For this review, take the finished solid that the model builds, in its own axes (mm). A direction names the side the tool comes from. Coordinates: 2 decimals unless noted, no trailing zeros. Loops run counter-clockwise (first coordinate to the right, second up) from the corner with the lowest first, then second, coordinate; pieces in that order, holes last. Notation, with made-up numbers: (54.5, 72) -> (112.5, 72) arc R16 ccw to (112.5, 100) -> close; hole circle Ø3 at (79.25, 32.5). An arc over 180 degrees is marked (long way). Use a Markdown table: item, result.
from build123d import *

# Parameters (mm, degrees)
F1_DEPTH = 225
F3_D     = 8
F5_D     = 5.9


with BuildPart() as f1:
    # F0 (on Front) → F1 (new body, symmetric)
    with BuildSketch(Plane.XZ):
        Polygon((-22.5, -22.5), (22.5, -22.5), (22.5, -18.5), (-18.5, -18.5), (-18.5, 22.5), (-22.5, 22.5), align=None)
    extrude(amount=F1_DEPTH, both=True)

    # F3 (through all)
    with Locations(Plane(origin=(-22.5, 0, 0), x_dir=(0, -1, 0), z_dir=(-1, 0, 0))):
        with Locations((-75, 12.5), (-85, -7.5), (-65, -7.5)):
            Hole(F3_D / 2)

    # F5 (through all)
    with Locations(Plane.XY.offset(-18.5)):
        with Locations((-13.5, -170), (16.5, -170), (16.5, -215), (-13.5, -215), (-13.5, 215), (16.5, 215), (16.5, 170), (-13.5, 170)):
            Hole(F5_D / 2)


solid = f1.part
(1) Mouldability with a two-part tool opening along Y and no side actions: class faces 1 (the face through (-20.47, 72.05, 15.2)), 2 (the face through (-20, -225, -10)), 3 (the face through (-18.5, -3, 2)) as pulls with the +Y half, pulls with the -Y half, needs draft (parallel to the pull), parting line crosses it, or undercut.
Found:
| item | result |
|---|---|
| face 1 | undercut |
| face 2 | pulls with the -Y half |
| face 3 | needs draft |
(2) Take a section at B-B on z = 12.5. Write out the cut boundary in (x, y).
Found:
| item | result |
|---|---|
| outline | (-22.5, -225) -> (-18.5, -225) -> (-18.5, 71) -> (-22.5, 71) -> close; (-22.5, 79) -> (-18.5, 79) -> (-18.5, 225) -> (-22.5, 225) -> close |
(3) Take a section at A-A on y = 75. Write out the cut boundary in (x, z).
Found:
| item | result |
|---|---|
| outline | (-22.5, -22.5) -> (22.5, -22.5) -> (22.5, -18.5) -> (-18.5, -18.5) -> (-18.5, 8.5) -> (-22.5, 8.5) -> close; (-22.5, 16.5) -> (-18.5, 16.5) -> (-18.5, 22.5) -> (-22.5, 22.5) -> close |
(4) Take a section at D-D on x = 9.5. Write out the cut boundary in (y, z), plus the area to 3 significant figures.
Found:
| item | result |
|---|---|
| outline | (-225, -22.5) -> (225, -22.5) -> (225, -18.5) -> (-225, -18.5) -> close |
| area | 1,800 mm^2 |
(5) For pin 1 Ø13 at (y, z) = (75, 12.5) entering from +X; pin 2 Ø9.5 at (x, y) = (16.5, 170) entering from +Z, all flat-tipped, find the tip position at first contact; note any pin that passes through.
Found:
| item | result |
|---|---|
| pin 1 | stops at x = -18.5 |
| pin 2 | stops at z = -18.5 |
(6) Take a section at C-C on z = -7.5. Write out the cut boundary in (x, y).
Found:
| item | result |
|---|---|
| outline | (-22.5, -225) -> (-18.5, -225) -> (-18.5, 61) -> (-22.5, 61) -> close; (-22.5, 69) -> (-18.5, 69) -> (-18.5, 81) -> (-22.5, 81) -> close; (-22.5, 89) -> (-18.5, 89) -> (-18.5, 225) -> (-22.5, 225) -> close |
(7) For line 1 along Y through (x, z) = (-13.5, -20.25); line 2 along X through (y, z) = (170, -20.55); line 3 along Z through (x, y) = (-20, 65), list the stretches that pass through material, from the lowest coordinate up.
Found:
| item | result |
|---|---|
| line 1 | y = -225 to -217.95, -212.05 to -172.95, -167.05 to 167.05, 172.95 to 212.05, 217.95 to 225 |
| line 2 | x = -22.5 to -16.45, -10.55 to 13.55, 19.45 to 22.5 |
| line 3 | z = -22.5 to -11.5, -3.5 to 22.5 |
(8) For faces 4 (the face through (2, -3, -18.5)), 5 (the face through (-20, 225, -10)), list the 3-axis set-ups (+Z, -Z, +X, -X, +Y, -Y) from which the entire face can be reached by the end or side of a thin tool; tool diameter is ignored.
Found:
| item | result |
|---|---|
| face 4 | +Z, +X, +Y, -Y |
| face 5 | +Z, -Z, +X, -X, +Y |
